Geometry check sheet. Reference: the model listing, model coordinates, mm. A direction names the side the tool comes from. Give positions to 0.01 mm unless a question says otherwise; leave off trailing zeros. Loops run counter-clockwise (first coordinate to the right, second up) from the corner with the lowest first, then second, coordinate; pieces in that order, holes last. Notation, with made-up numbers: (43, 15.5) -> (99, 15.5) arc R31 ccw to (99, 39.5) -> close; hole circle Ø9 at (23, 72). An arc over 180 degrees is marked (long way). Answer as a JSON object with one key per item and string values.
from build123d import *

# Parameters (mm, degrees)
F0_W     = 32
F0_H     = 32
F0_W_2   = 30
F0_H_2   = 30
F1_DEPTH = 30
F3_DEPTH = 50


with BuildPart() as f1:
    # F0 (on Top) → F1 (new body)
    with BuildSketch(Plane.XY):
        Rectangle(F0_W, F0_H)
        Rectangle(F0_W_2, F0_H_2, mode=Mode.SUBTRACT)
    extrude(amount=F1_DEPTH)

    # F2 (on face) → F3 (cut)
    with BuildSketch(Plane.XZ.offset(16)):
        with BuildLine():
            ThreePointArc((0, 12.5), (1.767767, 13.232233), (2.5, 15))
            ThreePointArc((2.5, 15), (-1.767767, 16.767767), (0, 12.5))
        make_face()
    extrude(amount=-F3_DEPTH, mode=Mode.SUBTRACT)


solid = f1.part
1) Section check B-B on y = -13. Record the cut outline in (x, z), plus the area to 3 significant figures.
Geometry check:
{"outline": "(-16, 0) -> (-15, 0) -> (-15, 30) -> (-16, 30) -> close; (15, 0) -> (16, 0) -> (16, 30) -> (15, 30) -> close", "area": "60.0 mm2"}
2) Material ranges on line 1 along X through (y, z) = (15.55, 15); line 2 along X through (y, z) = (-4.5, 8.5), recorded low to high. Write a range as from..to.
Geometry check:
{"line 1": "x = -16..-2.5, 2.5..16", "line 2": "x = -16..-15, 15..16"}
3) Depth check by flat-ended pin: P1, Ø6, axis at x = 0, z = 15, coming from the +Y side. Enter the tip coordinate at first touch or a pass-through.
Geometry check:
{"P1": "stops at y = 16"}
4) Tool access check on faces 1 (the face through (-4, 15, 15)), 2 (the face through (0, -16, 11)). Record the directions out of +Z, -Z, +X, -X, +Y, -Y that give a thin tool (end or side, any length) a straight path to the whole face; none if there is none.
Geometry check:
{"face 1": "+Z, -Z", "face 2": "+Z, -Z, +X, -X, -Y"}
5) Draft check along X on faces 3 (the face through (-1.3, -15.3, 30)), 4 (the face through (-16, 0, 15)), 5 (the face through (-4, -15, 15)). Enter one of: pulls with the +X half, pulls with the -X half, needs draft (parallel to the pull), parting line crosses it, or undercut.
Geometry check:
{"face 3": "needs draft", "face 4": "pulls with the -X half", "face 5": "undercut"}
6) Section check A-A on z = 21.75. Record the cut outline in (x, y), plus the area to 3 significant figures.
Geometry check:
{"outline": "(-16, -16) -> (16, -16) -> (16, 16) -> (-16, 16) -> close; hole (-15, -15) -> (15, -15) -> (15, 15) -> (-15, 15) -> close", "area": "124 mm2"}
7) Section check D-D on z = 16. Record the cut outline in (x, y), plus the area to 3 significant figures.
Geometry check:
{"outline": "(-16, -16) -> (-2.29, -16) -> (-2.29, -15) -> (-15, -15) -> (-15, 15) -> (-2.29, 15) -> (-2.29, 16) -> (-16, 16) -> close; (2.29, -16) -> (16, -16) -> (16, 16) -> (2.29, 16) -> (2.29, 15) -> (15, 15) -> (15, -15) -> (2.29, -15) -> close", "area": "115 mm2"}
